```python
from build123d import *

# Parameters (mm, degrees)
F1_DEPTH = 2.54
F2_R     = 1.4605
F3_DEPTH = 2.541
F5_DEPTH = 2.54
F4_R     = 1.27
F6_DEPTH = 25.4


with BuildPart() as f1:
    # F0 (on Top) → F1 (new body)
    with BuildSketch(Plane.XY):
        with BuildLine():
            Line((12.7, -50.8), (12.7, 50.8))
            ThreePointArc((12.7, 50.8), (0, 63.5), (-12.7, 50.8))
            Line((-12.7, 50.8), (-12.7, -50.8))
            ThreePointArc((-12.7, -50.8), (0, -63.5), (12.7, -50.8))
        make_face()
        with BuildLine():
            Line((4.318, -50.7966617284), (-4.318, -50.7966617284))
            ThreePointArc((-4.318, -50.7966617284), (-8.437248663, -52.5029103914), (-6.731, -48.3836617284))
            Line((-6.731, -48.3836617284), (-6.731, -39.7476617284))
            ThreePointArc((-6.731, -39.7476617284), (-8.437248663, -35.6284130654), (-4.318, -37.3346617284))
            Line((-4.318, -37.3346617284), (4.318, -37.3346617284))
            ThreePointArc((4.318, -37.3346617284), (6.731, -34.9216617284), (9.144, -37.3346617284))
            ThreePointArc((9.144, -37.3346617284), (8.437248663, -39.0409103914), (6.731, -39.7476617284))
            Line((6.731, -39.7476617284), (6.731, -48.3836617284))
            ThreePointArc((6.731, -48.3836617284), (8.437248663, -49.0904130654), (9.144, -50.7966617284))
            ThreePointArc((9.144, -50.7966617284), (6.731, -53.2096617284), (4.318, -50.7966617284))
        make_face(mode=Mode.SUBTRACT)
        with BuildLine():
            ThreePointArc((-6.731, -48.3836617284), (-5.024751337, -49.0904130654), (-4.318, -50.7966617284))
            Line((-4.318, -50.7966617284), (4.318, -50.7966617284))
            ThreePointArc((4.318, -50.7966617284), (5.024751337, -49.0904130654), (6.731, -48.3836617284))
            Line((6.731, -48.3836617284), (6.731, -39.7476617284))
            ThreePointArc((6.731, -39.7476617284), (5.024751337, -39.0409103914), (4.318, -37.3346617284))
            Line((4.318, -37.3346617284), (-4.318, -37.3346617284))
            ThreePointArc((-4.318, -37.3346617284), (-5.024751337, -39.0409103914), (-6.731, -39.7476617284))
            Line((-6.731, -39.7476617284), (-6.731, -48.3836617284))
        make_face()
    extrude(amount=F1_DEPTH)

    # F2 (on face) → F3 (cut, through all)
    with BuildSketch(Plane.XY.offset(2.54)):
        Circle(F2_R)
    extrude(amount=-F3_DEPTH, mode=Mode.SUBTRACT)

    # F4 (on face) → F5 (join, through all)
    with BuildSketch(Plane.XY.offset(2.54)):
        with BuildLine():
            ThreePointArc((12.7, 4.4121561861), (18.5710130473, 24.7321561861), (12.7, 45.0521561861))
            Line((12.7, 45.0521561861), (12.7, 4.4121561861))
        make_face()
        with BuildLine():
            Line((-12.7, 4.4121561861), (-12.7, 45.0521561861))
            ThreePointArc((-12.7, 45.0521561861), (-18.5710130473, 24.7321561861), (-12.7, 4.4121561861))
        make_face()
    extrude(amount=-F5_DEPTH)

    # F4 (on face) → F6 (cut)
    with BuildSketch(Plane.XY.offset(2.54)):
        Polygon((10.16, 4.4121561861), (10.16, 45.0521561861), (7.62, 45.0521561861), (7.62, 37.1781561861), (0, 37.1781561861), (-7.62, 37.1781561861), (-7.62, 45.0521561861), (-10.16, 45.0521561861), (-10.16, 4.4121561861), align=None)
        Polygon((7.62, 37.1781561861), (7.62, 45.0521561861), (-7.62, 45.0521561861), (-7.62, 37.1781561861), (0, 37.1781561861), align=None)
        with BuildLine():
            ThreePointArc((6.35, 50.6401561861), (6.7219743879, 49.742130574), (7.62, 49.3701561861))
            Line((7.62, 49.3701561861), (7.62, 50.6401561861))
            Line((7.62, 50.6401561861), (6.35, 50.6401561861))
        make_face()
        with BuildLine():
            Line((7.62, 50.6401561861), (7.62, 49.3701561861))
            ThreePointArc((7.62, 49.3701561861), (8.5180256121, 49.742130574), (8.89, 50.6401561861))
            Line((8.89, 50.6401561861), (7.62, 50.6401561861))
        make_face()
        with BuildLine():
            Line((7.62, 50.6401561861), (8.89, 50.6401561861))
            ThreePointArc((8.89, 50.6401561861), (7.62, 51.9101561861), (6.35, 50.6401561861))
            Line((6.35, 50.6401561861), (7.62, 50.6401561861))
        make_face()
        with BuildLine():
            ThreePointArc((-8.89, 50.6401561861), (-8.5180256121, 49.742130574), (-7.62, 49.3701561861))
            Line((-7.62, 49.3701561861), (-7.62, 50.6401561861))
            Line((-7.62, 50.6401561861), (-8.89, 50.6401561861))
        make_face()
        with BuildLine():
            Line((-7.62, 50.6401561861), (-7.62, 49.3701561861))
            ThreePointArc((-7.62, 49.3701561861), (-6.7219743879, 49.742130574), (-6.35, 50.6401561861))
            Line((-6.35, 50.6401561861), (-7.62, 50.6401561861))
        make_face()
        with BuildLine():
            Line((-8.89, 50.6401561861), (-7.62, 50.6401561861))
            Line((-7.62, 50.6401561861), (-6.35, 50.6401561861))
            ThreePointArc((-6.35, 50.6401561861), (-7.62, 51.9101561861), (-8.89, 50.6401561861))
        make_face()
        with Locations((-7.62, -1.1758438139)):
            Circle(F4_R)
        with Locations((7.62, -1.1758438139)):
            Circle(F4_R)
    extrude(amount=-F6_DEPTH, mode=Mode.SUBTRACT)


solid = f1.part
```
For this review, take the finished solid that the model builds, in its own axes (mm). A direction names the side the tool comes from. Coordinates: 2 decimals unless noted, no trailing zeros. Loops run counter-clockwise (first coordinate to the right, second up) from the corner with the lowest first, then second, coordinate; pieces in that order, holes last. Notation, with made-up numbers: (21, -4) -> (79, -4) arc R14 ccw to (79, 9) -> close; hole circle Ø2 at (40.25, 27.25). An arc over 180 degrees is marked (long way). Return JSON: item names as keys, results as strings. Group by question number.
(1) Consider section A-A, the plane y = 34.5. Give the boundary of the cut face in (x, z), plus the area to 3 significant figures.
(2) Consider section B-B, the plane z = 1.8. Count the separate pieces of the cut face and the enclosed holes in it, plus the area to 3 significant figures.
(3) For pin 1 Ø1.3 at (y, z) = (22, 2) entering from -X; pin 2 Ø1.3 at (y, z) = (-28.5, 2) entering from +X; pin 3 Ø0.8 at (y, z) = (-10, 1) entering from -X, all flat-tipped, find the tip position at first contact; note any pin that passes through.
(4) Consider section D-D, the plane x = 14. Give the boundary of the cut face in (y, z), plus the area to 3 significant figures.
(5) To check wall thickness, follow L1, parallel to Y at x = 0, z = 1.45; L2, parallel to Y at x = -1, z = 0.75; L3, parallel to Y at x = 7.62, z = 1.75. State the ranges of each line that lie inside material, in increasing order.
(6) Tool access review of faces 1 (the flat face through (12.7, 48, 1)), 2 (the flat face through (-12.7, 48, 1)), 3 (the flat face through (0, 4.412, 1)): name each direction out of +Z, -Z, +X, -X, +Y, -Y from which nothing blocks a thin tool from reaching the whole face with its end or side.
(7) Mouldability with a two-part tool opening along Y and no side actions: class faces 4 (the cylindrical face through (-0.279, -63.497, 1.252)), 5 (the flat face through (-12.7, -23, 1)), 6 (the flat face through (-10.16, 25, 1)) as pulls with the +Y half, pulls with the -Y half, needs draft (parallel to the pull), parting line crosses it, or undercut.
(8) Consider section C-C, the plane y = 55. Give the boundary of the cut face in (x, z).
Results below:
{
 "1": {"outline": "(-17.3, 0) -> (-10.16, 0) -> (-10.16, 2.54) -> (-17.3, 2.54) -> close; (10.16, 0) -> (17.3, 0) -> (17.3, 2.54) -> (10.16, 2.54) -> close", "area": "36.3 mm2"},
 "2": {"separate pieces": "1", "enclosed holes": "10", "area": "2,480 mm2"},
 "3": {"pin 1": "stops at x = -18.51", "pin 2": "stops at x = 12.7", "pin 3": "stops at x = -12.7"},
 "4": {"outline": "(6.64, 0) -> (42.83, 0) -> (42.83, 2.54) -> (6.64, 2.54) -> close", "area": "91.9 mm2"},
 "5": {"L1": "y = -63.5 to -1.46, 1.46 to 4.41, 45.05 to 63.5", "L2": "y = -63.46 to -1.06, 1.06 to 4.41, 45.05 to 63.46", "L3": "y = -60.96 to -53.04, -48.55 to -39.58, -35.09 to -2.45, 0.09 to 4.41, 45.05 to 49.37, 51.91 to 60.96"},
 "6": {"face 1": "+Z, -Z, +X, +Y", "face 2": "+Z, -Z, -X, +Y", "face 3": "+Z, -Z"},
 "7": {"face 4": "pulls with the -Y half", "face 5": "needs draft", "face 6": "undercut"},
 "8": {"outline": "(-11.99, 0) -> (11.99, 0) -> (11.99, 2.54) -> (-11.99, 2.54) -> close"}
}
